```python
from build123d import *

# Parameters (mm, degrees)
CUT_EXTRUDE_1_DEPTH      = 29.158391289
CUT_EXTRUDE_1_DEPTH_BACK = 29.158391289
SKETCH_2_R               = 15.051532373


with BuildPart() as part:
    # 草圖1 → 旋轉1 (revolve)
    with BuildSketch(Plane.XY, mode=Mode.PRIVATE) as revolve_1_sk:
        with BuildLine():
            ThreePointArc((6.5, -9), (6.125834261, -8.741421356), (6.235424869, -8.3))
            Line((6.235424869, -8.3), (6.1, -8.3))
            Line((6.1, -8.3), (6.1, -3.4))
            Line((6.1, -3.4), (5.75, -3.4))
            Line((5.75, -3.4), (5.75, 3.4))
            Line((5.75, 3.4), (6.1, 3.4))
            Line((6.1, 3.4), (6.1, 8.3))
            Line((6.1, 8.3), (6.235424869, 8.3))
            ThreePointArc((6.235424869, 8.3), (6.125834261, 8.741421356), (6.5, 9))
            Line((6.5, 9), (7.1, 9))
            Line((7.1, 9), (7.1, 12.5))
            Line((7.1, 12.5), (6.1, 12.5))
            Line((6.1, 12.5), (6.1, 19.792893219))
            Line((6.1, 19.792893219), (6.807106781, 20.5))
            Line((6.807106781, 20.5), (9.067157288, 20.5))
            Line((9.067157288, 20.5), (9.35, 20.217157288))
            Line((9.35, 20.217157288), (9.35, 18.782842712))
            Line((9.35, 18.782842712), (9.067157288, 18.5))
            Line((9.067157288, 18.5), (7.35, 18.5))
            Line((7.35, 18.5), (7.35, 17))
            Line((7.35, 17), (9.35, 17))
            Line((9.35, 17), (9.35, 15))
            Line((9.35, 15), (10, 14.35))
            Line((10, 14.35), (10, -14.35))
            Line((10, -14.35), (9.35, -15))
            Line((9.35, -15), (9.35, -17))
            Line((9.35, -17), (7.35, -17))
            Line((7.35, -17), (7.35, -18.5))
            Line((7.35, -18.5), (9.067157288, -18.5))
            Line((9.067157288, -18.5), (9.35, -18.782842712))
            Line((9.35, -18.782842712), (9.35, -20.217157288))
            Line((9.35, -20.217157288), (9.067157288, -20.5))
            Line((9.067157288, -20.5), (6.807106781, -20.5))
            Line((6.807106781, -20.5), (6.1, -19.792893219))
            Line((6.1, -19.792893219), (6.1, -12.5))
            Line((6.1, -12.5), (7.1, -12.5))
            Line((7.1, -12.5), (7.1, -9))
            Line((7.1, -9), (6.5, -9))
        make_face()
        Polygon((11.85, 10), (10, 10), (10, 6), (13.65, 6), (13.65, 9), align=None)
        Polygon((13.65, -6), (10, -6), (10, -10), (11.85, -10), (13.65, -9), align=None)
    revolve(revolve_1_sk.sketch.rotate(Axis((0, 26.248758247, 0), (0, -1, 0)), 90), axis=Axis((0, 26.248758247, 0), (0, -1, 0)))

    # 草圖2 → 除料-伸長1 (cut, two sides: drawn at the far end of the back side and taken through both)
    with BuildSketch(Plane(origin=(0, 0, 0), x_dir=(1, 0, 0), z_dir=(0, 1, 0)).offset(-CUT_EXTRUDE_1_DEPTH_BACK)):
        Circle(SKETCH_2_R)
        Polygon((13.856406461, 0), (6.92820323, 12), (-6.92820323, 12), (-13.856406461, 0), (-6.92820323, -12), (6.92820323, -12), align=None, mode=Mode.SUBTRACT)
    extrude(amount=CUT_EXTRUDE_1_DEPTH + CUT_EXTRUDE_1_DEPTH_BACK, mode=Mode.SUBTRACT)


solid = part.part
```
Geometry: final body of the model. Coordinates: model frame, mm. A direction names the side the tool comes from. Coordinates: 2 decimals unless noted, no trailing zeros. Order: outer loops, then holes, each group sorted by start corner. A loop starts at its lowest first (then second) coordinate and runs counter-clockwise, first axis right, second up. Notation, with made-up numbers: M 78.5,-20.5 L 101.5,-20.5 A8 ccw 101.5,-6.5 Z; hole C 30.25,-30 d6. An arc over 180 degrees is marked long. Answer in a Markdown table with one row per item. Add a question column.
Q1. Section query B-B on x = -8. Count the separate pieces of the cut face and the enclosed holes in it, and give its area (3 significant figures).
Q2. Line query: L1, parallel to Y at x = 0.75, z = 8.75; L2, parallel to X at y = -0.25, z = 0; L3, parallel to Y at x = 4.5, z = 5.25. Output: solid intervals per line, ascending.
Q3. Section query A-A on y = -16. Return the cut outline in (x, z), and give its area (3 significant figures).
Q4. Reachability of faces 1 (the flat face through (3, -10, 10)), 2 (the cylindrical face through (0, 0, -10)), 3 (the cylindrical face through (8.295, 19.49, 4.314)) from +Z, -Z, +X, -X, +Y, -Y: full face, straight path, thin tool, end or side. Return the list, or none.
Q5. Mould query, pull axis X, two halves, no side actions, for faces 4 (the flat face through (0, -8, 12)), 5 (the flat face through (6, -9, 3)), 6 (the cylindrical face through (7.175, -17.76, -1.593)). Classes: released by +X, released by -X, zero draft, split by the parting line, or undercut.
Q6. Contact query for flat-ended pins moving along their axis: P1, Ø8, axis at y = 1, z = 7.5, coming from the +X side; P2, Ø12, axis at x = -9.5, z = -6.5, coming from the -Y side; P3, Ø4, axis at x = 6, y = -14.5, coming from the +Z side; P4, Ø3, axis at y = 3.5, z = -8, coming from the -X side. Output: stop coordinate, or through.
Completed:
| question | item | result |
|---|---|---|
| 1 | separate pieces | 3 |
| 1 | enclosed holes | 0 |
| 1 | area | 500 mm2 |
| 2 | L1 | y = -20.5 to -18.5, -17 to 17, 18.5 to 20.5 |
| 2 | L2 | x = -10 to -5.75, 5.75 to 10 |
| 2 | L3 | y = -20.5 to -12.5, -9 to 9, 12.5 to 20.5 |
| 3 | outline | C 0,0 d18.7; hole C 0,0 d12.2 |
| 3 | area | 158 mm2 |
| 4 | face 1 | -Y |
| 4 | face 2 | none |
| 4 | face 3 | +Y |
| 5 | face 4 | zero draft |
| 5 | face 5 | undercut |
| 5 | face 6 | split by the parting line |
| 6 | P1 | stops at x = 9.37 |
| 6 | P2 | stops at y = -20.5 |
| 6 | P3 | stops at z = 9.16 |
| 6 | P4 | stops at x = -7.6 |
